Source: CAD feature listing. Evaluate the final solid. Frame: model axes, mm. Give positions to 0.01 mm unless a question says otherwise; leave off trailing zeros. Loops run counter-clockwise (first coordinate to the right, second up) from the corner with the lowest first, then second, coordinate; pieces in that order, holes last. Notation, with made-up numbers: (-30.5, 62) -> (-14.5, 62) arc R18 ccw to (-14.5, 66) -> close; hole circle Ø3 at (42, 21.5). An arc over 180 degrees is marked (long way). Put each result on its own line as item: value.
```python
from build123d import *

# Parameters (mm, degrees)
F0_R     = 1.25
F0_W     = 8.466002
F0_H     = 8.417533
F1_DEPTH = 2


with BuildPart() as f1:
    # F0 (on Top) → F1 (new body)
    with BuildSketch(Plane.XY):
        with BuildLine():
            Line((19.377316, 48.371452), (12.511831, 48.371452))
            Line((12.511831, 48.371452), (11.281675, 48.362336))
            Line((11.281675, 48.362336), (10.424009, 49.616981))
            Line((10.424009, 49.616981), (8.498245, 49.616981))
            Line((8.498245, 49.616981), (8.498245, 46.11221))
            Line((8.498245, 46.11221), (8.592918, 24.0495))
            ThreePointArc((8.592918, 24.0495), (8.964934, 22.283302), (10.245487, 21.011281))
            ThreePointArc((10.245487, 21.011281), (11.017389, 20.275696), (11.301618, 19.248014))
            Line((11.301618, 19.248014), (11.301618, 17.655057))
            ThreePointArc((11.301618, 17.655057), (11.147379, 16.705509), (10.700523, 15.853599))
            ThreePointArc((10.700523, 15.853599), (10.34255, 15.063964), (10.352377, 14.197032))
            Line((10.352377, 14.197032), (13.388781, 1.218066))
            ThreePointArc((13.388781, 1.218066), (13.926743, 0.254704), (14.893698, -0.276774))
            Line((14.893698, -0.276774), (17.223874, -0.805427))
            ThreePointArc((17.223874, -0.805427), (17.646499, -0.708531), (17.834499, -0.317819))
            Line((17.834499, -0.317819), (17.834499, 5.715386))
            ThreePointArc((17.834499, 5.715386), (18.0225, 6.106098), (18.445124, 6.202995))
            Line((18.445124, 6.202995), (21.28958, 5.557665))
            ThreePointArc((21.28958, 5.557665), (21.732081, 5.5081), (22.174581, 5.557665))
            Line((22.174581, 5.557665), (25.019037, 6.202995))
            ThreePointArc((25.019037, 6.202995), (25.441662, 6.106098), (25.629662, 5.715386))
            Line((25.629662, 5.715386), (25.629662, -0.317819))
            ThreePointArc((25.629662, -0.317819), (25.817662, -0.708531), (26.240287, -0.805427))
            Line((26.240287, -0.805427), (28.570463, -0.276774))
            ThreePointArc((28.570463, -0.276774), (29.537418, 0.254704), (30.07538, 1.218066))
            Line((30.07538, 1.218066), (33.111785, 14.197032))
            ThreePointArc((33.111785, 14.197032), (33.121611, 15.063964), (32.763638, 15.853599))
            ThreePointArc((32.763638, 15.853599), (32.316782, 16.705509), (32.162543, 17.655057))
            Line((32.162543, 17.655057), (32.162543, 19.248014))
            ThreePointArc((32.162543, 19.248014), (32.446773, 20.275696), (33.218674, 21.011281))
            ThreePointArc((33.218674, 21.011281), (34.499227, 22.283302), (34.871243, 24.0495))
            Line((34.871243, 24.0495), (34.965916, 46.11221))
            Line((34.965916, 46.11221), (34.965916, 49.616981))
            Line((34.965916, 49.616981), (33.040153, 49.616981))
            Line((33.040153, 49.616981), (32.182486, 48.362336))
            Line((32.182486, 48.362336), (30.95233, 48.371452))
            Line((30.95233, 48.371452), (24.086845, 48.371452))
            ThreePointArc((24.086845, 48.371452), (21.732081, 50.726217), (19.377316, 48.371452))
        make_face()
        with Locations((15.982081, 3.955105)):
            Circle(F0_R, mode=Mode.SUBTRACT)
        with Locations((11.732081, 23.788427)):
            Circle(F0_R, mode=Mode.SUBTRACT)
        with Locations((27.482081, 3.955105)):
            Circle(F0_R, mode=Mode.SUBTRACT)
        with Locations((31.732081, 23.788427)):
            Circle(F0_R, mode=Mode.SUBTRACT)
        with Locations((11.732081, 43.788427)):
            Circle(F0_R, mode=Mode.SUBTRACT)
        with Locations((18.679423, 39.579661)):
            Rectangle(F0_W, F0_H, mode=Mode.SUBTRACT)
        with Locations((21.732081, 48.371452)):
            Circle(F0_R, mode=Mode.SUBTRACT)
        with Locations((31.732081, 43.788427)):
            Circle(F0_R, mode=Mode.SUBTRACT)
    extrude(amount=F1_DEPTH)


solid = f1.part
```
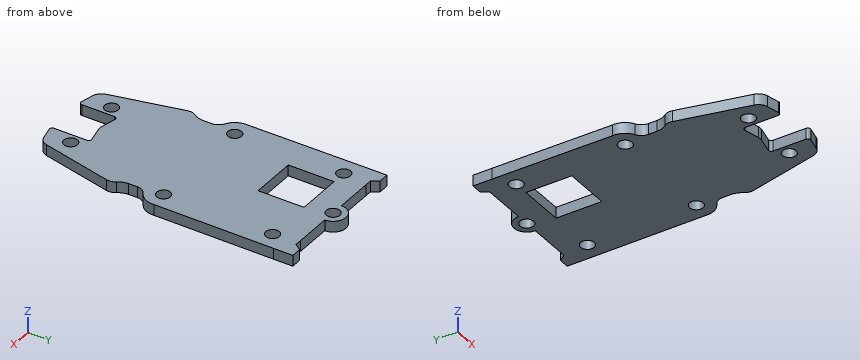
(1) Section D-D on y = 15. Return loops of the section in (x, z), then the cut area to 3 significant figures.
Calculated:
outline: (10.33, 0) -> (33.13, 0) -> (33.13, 2) -> (10.33, 2) -> close
area: 45.6 mm²
(2) Section A-A on x = 16.75. Return loops of the section in (y, z).
Calculated:
outline: (-0.7, 0) -> (2.97, 0) -> (2.97, 2) -> (-0.7, 2) -> close; (4.94, 0) -> (35.37, 0) -> (35.37, 2) -> (4.94, 2) -> close; (43.79, 0) -> (48.37, 0) -> (48.37, 2) -> (43.79, 2) -> close
(3) Section B-B on x = 27.25. Return loops of the section in (y, z).
Calculated:
outline: (-0.58, 0) -> (2.73, 0) -> (2.73, 2) -> (-0.58, 2) -> close; (5.18, 0) -> (48.37, 0) -> (48.37, 2) -> (5.18, 2) -> close
(4) First-contact query: P1, Ø0.6, axis at x = 26.5, z = 0.5, coming from the +Y side; P2, Ø0.6, axis at x = 18.5, z = 1.5, coming from the -Y side; P3, Ø0.5, axis at y = 18.5, z = 1, coming from the +X side; P4, Ø1.5, axis at x = 11.73, y = 43.79, coming from the -Z side. Flat tips, straight axial feed; report the tip coordinate or a pass-through.
Calculated:
P1: stops at y = 48.37
P2: stops at y = 6.12
P3: stops at x = 32.16
P4: passes through
(5) Section C-C on z = 1. Give the number of separate pieces and of enclosed holes in the cut face, then the cut area to 3 significant figures.
Calculated:
separate pieces: 1
enclosed holes: 8
area: 1,010 mm²
(6) Line query: probe 1 along Y at (x, z) = (21.75, 1.8); probe 2 along Y at (x, z) = (17, 1.45); probe 3 along X at (y, z) = (43, 0.65). Output: solid intervals per line, ascending. Write a range as from..to.
Calculated:
probe 1: y = 5.51..35.37, 43.79..47.12, 49.62..50.73
probe 2: y = -0.75..3.23, 4.68..35.37, 43.79..48.37
probe 3: x = 8.51..10.76, 12.7..14.45, 22.91..30.76, 32.7..34.95
